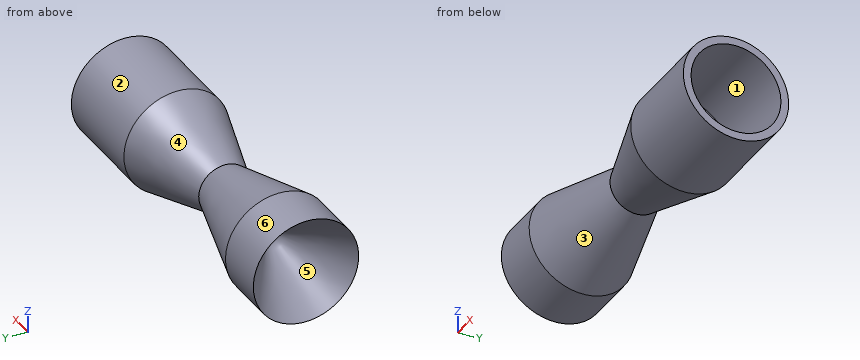
```python
from build123d import *

# Parameters (mm, degrees)
F2_T = -2.54


with BuildPart() as f1:
    # F0 (on Front) → F1 (revolve)
    with BuildSketch(Plane.XZ):
        Polygon((0, 8.3979964256), (-32.5231477618, 17.2540657222), (-49.3191406131, 17.2540657222), (-25.4993699491, 0), (60.6182664633, 0), (60.6182664633, 17.2540657222), (28.8585666567, 17.2540657222), align=None)
    revolve(axis=Axis((17.5594482571, 0, 0), (-1, 0, 0)))

    # F2
    f2_openings = [f1.faces().sort_by_distance(p)[0] for p in [
        (60.618266, 0, 0),
    ]]
    offset(amount=F2_T, openings=f2_openings, kind=Kind.INTERSECTION)


solid = f1.part
```
Here's how the part is built. I have some questions about the finished solid (model axes, mm). Face numbers are marked on the shaded views. A direction names the side the tool comes from. Coordinates: 2 decimals unless noted, no trailing zeros. Order: outer loops, then holes, each group sorted by start corner. A loop starts at its lowest first (then second) coordinate and runs counter-clockwise, first axis right, second up.
Item 1: Thinking about a two-plate mould opening in X: for the marked faces 4, 5 and 6, which applies, pulls with the +X half, pulls with the -X half, needs draft (parallel to the pull), parting line crosses it, or undercut?
Response values:
face 4: undercut
face 5: pulls with the -X half
face 6: needs draft
Item 2: If we section it at A-A, the plane y = -9.5: Give the number of separate pieces and of enclosed holes in the cut face, then the cut area to 3 significant figures.
Response values:
separate pieces: 2
enclosed holes: 1
area: 862 mm2
Item 3: I need wall thicknesses on probe 1 along Y at (x, z) = (43, 0); probe 2 along Y at (x, z) = (-35, 0); probe 3 along Z at (x, y) = (0, 1.5). Which ranges of each line are inside material? Lowest first, please.
Response values:
probe 1: y = -17.25 to -14.71, 14.71 to 17.25
probe 2: y = -17.25 to -14.71, -10.02 to -6.88, 6.88 to 10.02, 14.71 to 17.25
probe 3: z = -8.26 to -5.57, 5.57 to 8.26
Item 4: Which directions (+Z, -Z, +X, -X, +Y, -Y) give clear straight access to the entire face, cutting with the end or side of a thin tool? Please do the marked faces 1, 2 and 3.
Response values:
face 1: +X
face 2: +X, -X
face 3: none
Item 5: I'm going to push flat-ended pins straight in: pin 1 Ø2 at (x, y) = (-29.5, -4.5) entering from -Z; pin 2 Ø1 at (x, y) = (43.5, 2) entering from +Z; pin 3 Ø1.5 at (x, y) = (22.5, 0.5) entering from +Z. Where does each tip first touch, or does it pass through?
Response values:
pin 1: stops at z = -16.19
pin 2: stops at z = 17.19
pin 3: stops at z = 15.53
Item 6: If we section it at D-D, the plane x = 43: List the corners of the cut face in (y, z) for me, then the cut area to 3 significant figures.
Response values:
outline: circle Ø34.51 at (0, 0); hole circle Ø29.43 at (0, 0)
area: 255 mm2
Item 7: If we section it at C-C, the plane x = -19: List the corners of the cut face in (y, z) for me.
Response values:
outline: circle Ø27.14 at (0, 0); hole circle Ø21.88 at (0, 0)
